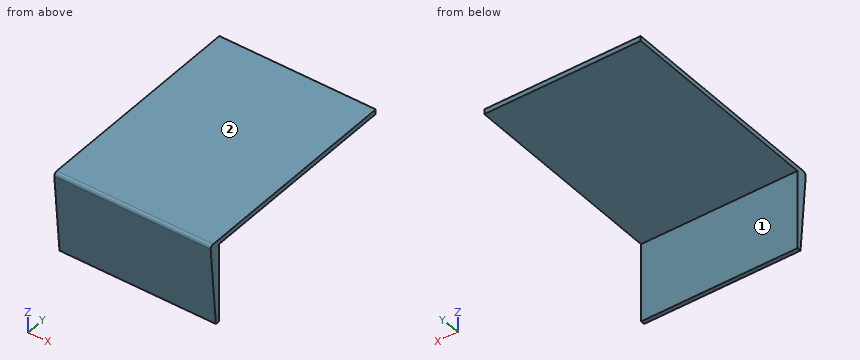
```python
from build123d import *

# Parameters (mm, degrees)
F1_DEPTH = 609.6


with BuildPart() as f1:
    # F0 (on Right) → F1 (new body)
    with BuildSketch(Plane.YZ):
        with BuildLine():
            Line((0, -307.975), (0, 0))
            Line((0, 0), (812.8, 0))
            Line((812.8, 0), (812.8, 19.05))
            Line((812.8, 19.05), (-29.861867, 19.05))
            ThreePointArc((-29.861867, 19.05), (-39.231667, 15.255664), (-42.8625, 5.821301))
            Line((-42.8625, 5.821301), (-15.875, -307.975))
            Line((-15.875, -307.975), (0, -307.975))
        make_face()
    extrude(amount=F1_DEPTH)


solid = f1.part
```
The listing builds one solid part. Answer for the finished solid, in the listing's coordinates (mm). Face numbers are marked on the shaded views. A direction names the side the tool comes from. Give positions to 0.01 mm unless a question says otherwise; leave off trailing zeros. Order: outer loops, then holes, each group sorted by start corner. A loop starts at its lowest first (then second) coordinate and runs counter-clockwise, first axis right, second up. Notation, with made-up numbers: (5, 23) -> (64, 23) arc R30 ccw to (64, 60) -> close; hole circle Ø5 at (65, -17.5). An arc over 180 degrees is marked (long way). Answer as a JSON object with one key per item and string values. Group by question number.
Item 1: The part is cut by section B-B on y = 479. Write down the section's boundary in (x, z), and give its area (3 significant figures).
Item 2: A tool of negligible diameter and unlimited length cuts with its end or side. For the marked faces 1 and 2, from which of +Z, -Z, +X, -X, +Y, -Y can it reach the whole face along a straight path? Write none if from no direction.
Item 3: Flat-ended cylindrical pins translate along their axes: pin 1 (1 mm diameter, centred on x = 481.5, y = 451, fed in from +Z); pin 2 (1 mm diameter, centred on x = 278.5, y = 96, fed in from -Z); pin 3 (8 mm diameter, centred on x = 222.5, y = 103, fed in from +Z). Find the tip coordinate at first contact, or state that the pin passes through.
Item 4: Consider L1, parallel to Z at x = 477.5, y = 166; L2, parallel to Y at x = 121.5, z = -170.5; L3, parallel to Y at x = 26.5, z = -254.5. Determine where each line is inside the solid, lowest interval first. Write a range as from..to.
Item 5: The part is cut by section C-C on z = -94.5. Write down the section's boundary in (x, y), and give its area (3 significant figures).
Result set:
{
 "1": {"outline": "(0, 0) -> (609.6, 0) -> (609.6, 19.05) -> (0, 19.05) -> close", "area": "11,600 mm²"},
 "2": {"face 1": "-Z, +X, -X, +Y", "face 2": "+Z, +X, -X, +Y, -Y"},
 "3": {"pin 1": "z = 19.05", "pin 2": "z = 0", "pin 3": "z = 19.05"},
 "4": {"L1": "0..19.05", "L2": "-27.7..0", "L3": "-20.47..0"},
 "5": {"outline": "(0, -34.23) -> (609.6, -34.23) -> (609.6, 0) -> (0, 0) -> close", "area": "20,900 mm²"}
}
